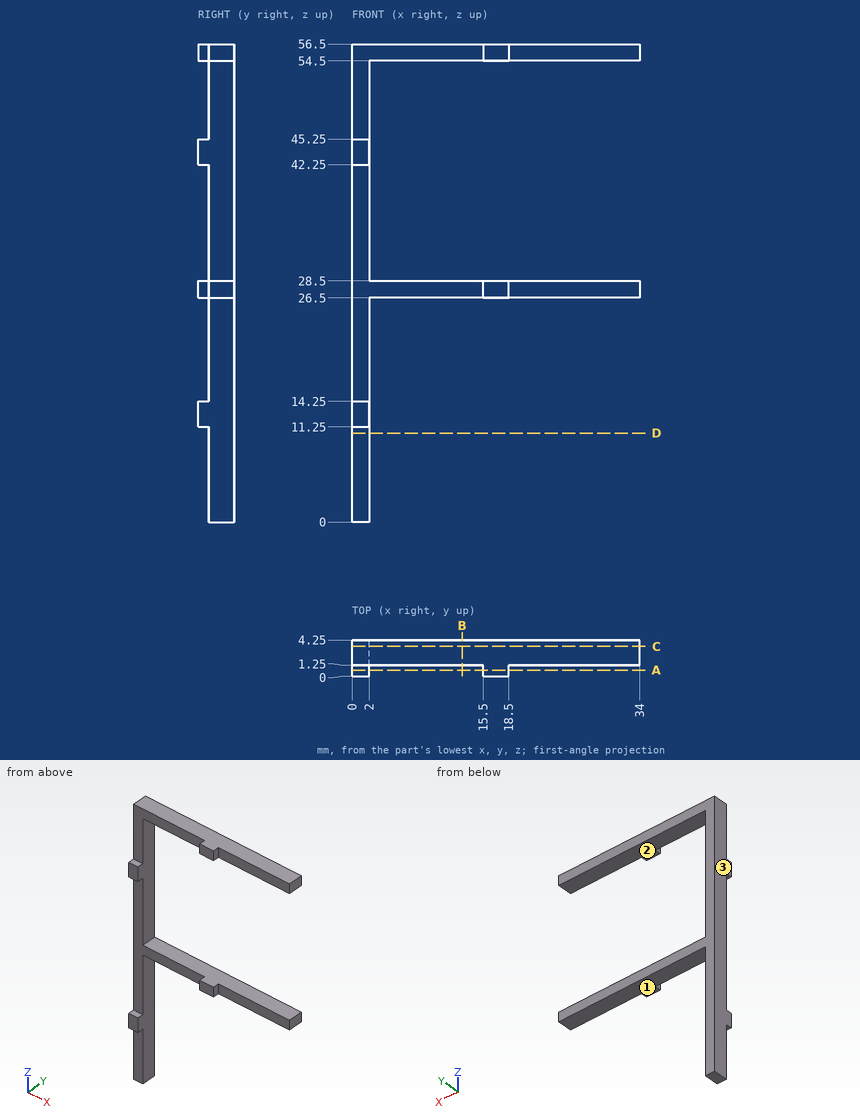
Input: dimensioned drawing with shaded views. Units: mm. Origin: part minimum x, y, z. A direction names the side the tool comes from. Give positions to 0.01 mm unless a question says otherwise; leave off trailing zeros. Loops run counter-clockwise (first coordinate to the right, second up) from the corner with the lowest first, then second, coordinate; pieces in that order, holes last. Notation, with made-up numbers: (40, 31) -> (63, 31) arc R6 cw to (63, 36) -> close; hole circle Ø3 at (-5.5, 34). An arc over 180 degrees is marked (long way). Use a Markdown table: item, result. Add a question column.
1) Section query D-D, the plane z = 10.5. Return the cut outline in (x, y).
2) Section query A-A, the plane y = 0.7. Return the cut outline in (x, z).
3) Section query B-B, the plane x = 13. Return the cut outline in (y, z), then the cut area to 3 significant figures.
4) Section query C-C, the plane y = 3.5. Return the cut outline in (x, z), then the cut area to 3 significant figures.
5) First-contact query: pin 1 (1 mm diameter, centred on x = 27.5, z = 55.5, fed in from -Y); pin 2 (1.3 mm diameter, centred on x = 19.5, y = 1.5, fed in from -Z); pin 3 (1.3 mm diameter, centred on y = 2.5, z = 35.5, fed in from +X). Flat tips, straight axial feed; report the tip coordinate or a pass-through.
6) Line query: line 1 along Z through (x, y) = (2.5, 1.6); line 2 along X through (y, z) = (2.3, 50.5). Output: solid intervals per line, ascending. Write a range as [from, to].
7) Reachability of the marked faces 1, 2 and 3 from +Z, -Z, +X, -X, +Y, -Y: full face, straight path, thin tool, end or side. Return the list, or none.
Numbers:
| question | item | result |
|---|---|---|
| 1 | outline | (0, 1.25) -> (2, 1.25) -> (2, 4.25) -> (0, 4.25) -> close |
| 2 | outline | (0, 11.25) -> (2, 11.25) -> (2, 14.25) -> (0, 14.25) -> close; (0, 42.25) -> (2, 42.25) -> (2, 45.25) -> (0, 45.25) -> close; (15.5, 26.5) -> (18.5, 26.5) -> (18.5, 28.5) -> (15.5, 28.5) -> close; (15.5, 54.5) -> (18.5, 54.5) -> (18.5, 56.5) -> (15.5, 56.5) -> close |
| 3 | outline | (1.25, 26.5) -> (4.25, 26.5) -> (4.25, 28.5) -> (1.25, 28.5) -> close; (1.25, 54.5) -> (4.25, 54.5) -> (4.25, 56.5) -> (1.25, 56.5) -> close |
| 3 | area | 12.0 mm2 |
| 4 | outline | (0, 0) -> (2, 0) -> (2, 26.5) -> (34, 26.5) -> (34, 28.5) -> (2, 28.5) -> (2, 54.5) -> (34, 54.5) -> (34, 56.5) -> (0, 56.5) -> close |
| 4 | area | 241 mm2 |
| 5 | pin 1 | stops at y = 1.25 |
| 5 | pin 2 | stops at z = 26.5 |
| 5 | pin 3 | stops at x = 2 |
| 6 | line 1 | z = [26.5, 28.5], [54.5, 56.5] |
| 6 | line 2 | x = [0, 2] |
| 7 | face 1 | -Z, +X, +Y, -Y |
| 7 | face 2 | +X, +Y, -Y |
| 7 | face 3 | +Z, -Z, -X, +Y, -Y |
